```python
from build123d import *

# Parameters (mm, degrees)
F1_DEPTH  = 27
F3_DEPTH  = 24
F5_DEPTH  = 3
F4_R      = 3.4
F6_DEPTH  = 3
F8_DEPTH  = 3
F9_R      = 3
F10_R     = 3.75
F11_DEPTH = 3


with BuildPart() as f1:
    # F0 (on Top) → F1 (new body)
    with BuildSketch(Plane.XY):
        with BuildLine():
            ThreePointArc((25, 15), (22.071068, 22.071068), (15, 25))
            Line((15, 25), (-15, 25))
            ThreePointArc((-15, 25), (-22.071068, 22.071068), (-25, 15))
            Line((-25, 15), (-25, -15))
            ThreePointArc((-25, -15), (-22.071068, -22.071068), (-15, -25))
            Line((-15, -25), (15, -25))
            ThreePointArc((15, -25), (22.071068, -22.071068), (25, -15))
            Line((25, -15), (25, 15))
        make_face()
    extrude(amount=F1_DEPTH)

    # F2 (on face) → F3 (cut)
    with BuildSketch(Plane.XY.offset(27)):
        with BuildLine():
            ThreePointArc((22.5, 14.5), (20.156854, 20.156854), (14.5, 22.5))
            Line((14.5, 22.5), (-14.5, 22.5))
            ThreePointArc((-14.5, 22.5), (-20.156854, 20.156854), (-22.5, 14.5))
            Line((-22.5, 14.5), (-22.5, -14.5))
            ThreePointArc((-22.5, -14.5), (-20.156854, -20.156854), (-14.5, -22.5))
            Line((-14.5, -22.5), (14.5, -22.5))
            ThreePointArc((14.5, -22.5), (20.156854, -20.156854), (22.5, -14.5))
            Line((22.5, -14.5), (22.5, 14.5))
        make_face()
    extrude(amount=-F3_DEPTH, mode=Mode.SUBTRACT)

    # F4 (on face) → F5 (cut)
    with BuildSketch(Plane.XY.offset(3)):
        with BuildLine():
            ThreePointArc((6, 3), (5.12132, 5.12132), (3, 6))
            Line((3, 6), (-3, 6))
            ThreePointArc((-3, 6), (-5.12132, 5.12132), (-6, 3))
            Line((-6, 3), (-6, -3))
            ThreePointArc((-6, -3), (-5.12132, -5.12132), (-3, -6))
            Line((-3, -6), (3, -6))
            ThreePointArc((3, -6), (5.12132, -5.12132), (6, -3))
            Line((6, -3), (6, 3))
        make_face()
    extrude(amount=-F5_DEPTH, mode=Mode.SUBTRACT)

    # F4 (on face) → F6 (cut)
    with BuildSketch(Plane.XY.offset(3)):
        with BuildLine():
            ThreePointArc((6, 3), (5.12132, 5.12132), (3, 6))
            Line((3, 6), (-3, 6))
            ThreePointArc((-3, 6), (-5.12132, 5.12132), (-6, 3))
            Line((-6, 3), (-6, -3))
            ThreePointArc((-6, -3), (-5.12132, -5.12132), (-3, -6))
            Line((-3, -6), (3, -6))
            ThreePointArc((3, -6), (5.12132, -5.12132), (6, -3))
            Line((6, -3), (6, 3))
        make_face()
        with Locations((0, 12)):
            Circle(F4_R)
    extrude(amount=-F6_DEPTH, mode=Mode.SUBTRACT)

    # F7 (on face) → F8 (cut)
    with BuildSketch(Plane(origin=(0, 25, 0), x_dir=(-1, 0, 0), z_dir=(0, 1, 0))):
        with BuildLine():
            Line((-3, 21), (3, 21))
            ThreePointArc((3, 21), (5.12132, 21.87868), (6, 24))
            Line((6, 24), (6, 27))
            Line((6, 27), (-6, 27))
            Line((-6, 27), (-6, 24))
            ThreePointArc((-6, 24), (-5.12132, 21.87868), (-3, 21))
        make_face()
    extrude(amount=-F8_DEPTH, mode=Mode.SUBTRACT)

    # F9
    f9_edges = [f1.edges().sort_by_distance(p)[0] for p in [
        (0, 25, 0),
    ]]
    fillet(f9_edges, radius=F9_R)

    # F10 (on face) → F11 (cut)
    with BuildSketch(Plane.YZ.offset(25)):
        with Locations((0, 14.75)):
            Circle(F10_R)
    extrude(amount=-F11_DEPTH, mode=Mode.SUBTRACT)


solid = f1.part
```
Part model, mm, in its own coordinate system. A direction names the side the tool comes from. Give positions to 0.01 mm unless a question says otherwise; leave off trailing zeros. Write each loop counter-clockwise with the first axis right and the second up, starting at its lowest first coordinate (ties: lowest second). Pieces come first, ordered by that corner, then holes. Notation, with made-up numbers: M 16.25,81.5 L 31.25,81.5 A28 cw 31.25,112.5 Z; hole C 15,45 d3. An arc over 180 degrees is marked long. Use CSV: the item, a comma, the result in double quotes.
Item 1: Drill centre lines: probe 1 along Y at (x, z) = (-2, 11.5); probe 2 along Y at (x, z) = (0, 2.25). Where is each one in solid material? Low to high.
Taken from the geometry:
probe 1,"y = -25 to -22.5, 22.5 to 25"
probe 2,"y = -24.9 to -6, 6 to 8.6, 15.4 to 24.9"
Item 2: Pin check, flat tips, straight feed: P1, Ø2.5, axis at y = 1, z = 2, coming from the -X side; P2, Ø0.9, axis at x = 0.5, z = 1.5, coming from the +Y side; P3, Ø2, axis at y = 23.5, z = 25, coming from the +X side; P4, Ø3, axis at y = 23.5, z = 25.5, coming from the -X side. Stop position of each tip, or through.
Taken from the geometry:
P1,"stops at x = -25"
P2,"stops at y = 24.81"
P3,"stops at x = 21.61"
P4,"stops at x = -22.14"
Item 3: Slice it at A-A on y = 12. Write the cut outline in (x, z), plus the area to 3 significant figures.
Taken from the geometry:
outline,"M -25,3 A3 ccw -22,0 L -3.4,0 L -3.4,3 L -22.5,3 L -22.5,27 L -25,27 Z; M 3.4,0 L 22,0 A3 ccw 25,3 L 25,27 L 22.5,27 L 22.5,3 L 3.4,3 Z"
area,"246 mm²"
Item 4: Slice it at C-C on y = 0. Write the cut outline in (x, z), plus the area to 3 significant figures.
Taken from the geometry:
outline,"M -25,3 A3 ccw -22,0 L -6,0 L -6,3 L -22.5,3 L -22.5,27 L -25,27 Z; M 6,0 L 22,0 A3 ccw 25,3 L 25,11 L 22.5,11 L 22.5,3 L 6,3 Z; M 22.5,18.5 L 25,18.5 L 25,27 L 22.5,27 Z"
area,"211 mm²"
Item 5: Slice it at D-D on x = 0. Write the cut outline in (y, z), plus the area to 3 significant figures.
Taken from the geometry:
outline,"M -25,3 A3 ccw -22,0 L -6,0 L -6,3 L -22.5,3 L -22.5,27 L -25,27 Z; M 6,0 L 8.6,0 L 8.6,3 L 6,3 Z; M 15.4,0 L 22,0 A3 ccw 25,3 L 25,21 L 22.5,21 L 22.5,3 L 15.4,3 Z"
area,"195 mm²"
Item 6: Which spindle directions (+Z, -Z, +X, -X, +Y, -Y) get a long thin tool onto all of the face, cutting with end or side? Do faces 1 (the face through (0, 22.5, 15)), 2 (the face through (0, 24, 21)), 3 (the face through (-6, 0, 2)). Say none if no direction does.
Taken from the geometry:
face 1,"+Z"
face 2,"+Z, +Y"
face 3,"+Z, -Z"
Item 7: Slice it at B-B on z = 14.75. Write the cut outline in (x, y), plus the area to 3 significant figures.
Taken from the geometry:
outline,"M -25,-15 A10 ccw -15,-25 L 15,-25 A10 ccw 25,-15 L 25,-3.75 L 22.5,-3.75 L 22.5,-14.5 A8 cw 14.5,-22.5 L -14.5,-22.5 A8 cw -22.5,-14.5 L -22.5,14.5 A8 cw -14.5,22.5 L 14.5,22.5 A8 cw 22.5,14.5 L 22.5,3.75 L 25,3.75 L 25,15 A10 ccw 15,25 L -15,25 A10 ccw -25,15 Z"
area,"425 mm²"
Item 8: Pull direction Y, two halves, no side cores. Call faces 4 (the face through (22.15, 21.99, 14.83)), 5 (the face through (5.14, 23.77, 21.9)), 6 (the face through (5.1, -5.14, 1.52)): +Y half, -Y half, draft (parallel to the pull), parting line (faces both ways), or undercut.
Taken from the geometry:
face 4,"+Y half"
face 5,"draft"
face 6,"undercut"
